Source: three-view drawing plus pictorial views. Frame: mm from the lowest corner of the part. A direction names the side the tool comes from. Round coordinates to 2 decimals unless told otherwise and drop trailing zeros. Order: outer loops, then holes, each group sorted by start corner. A loop starts at its lowest first (then second) coordinate and runs counter-clockwise, first axis right, second up. Notation, with made-up numbers: (-18.5, 49.25) -> (28.5, 49.25) arc R21 cw to (28.5, 70.25) -> close; hole circle Ø5 at (6, 29.5). An arc over 180 degrees is marked (long way). Answer as CSV lines item,"result". Start each with the question number.
1) Section query A-A, the plane y = 78.5. Output: boundary loops of the cut face in (x, z).
2) Section query D-D, the plane z = 10. State how many separate pieces and enclosed holes the cut face has, and give its area (3 significant figures).
3) Section query C-C, the plane y = 61. Output: boundary loops of the cut face in (x, z), and give its area (3 significant figures).
4) Line query: L1, parallel to Z at x = 33.5, y = 3; L2, parallel to Z at x = 113.7, y = 78.5; L3, parallel to X at y = 45.5, z = 13.25. Output: solid intervals per line, ascending.
5) Access query for the marked faces 1, 2, 3 and 4. Directions: +Z, -Z, +X, -X, +Y, -Y. A direction counts if a zero-diameter tool reaches every point of the face in a straight line with its end or side. Return the directions, or none.
6) First-contact query: P1, Ø6, axis at x = 9.5, z = 10, coming from the -Y side; P2, Ø3.5, axis at y = 12.5, z = 10.5, coming from the +X side; P3, Ø3.5, axis at x = 83.5, z = 15, coming from the +Y side. Flat tips, straight axial feed; report the tip coordinate or a pass-through.
7) Section query B-B, the plane x = 33.5. Output: boundary loops of the cut face in (y, z).
8) Mould query, pull axis X, two halves, no side actions, for the marked faces 5, 6, 7 and 8. Classes: +X half, -X half, draft (parallel to the pull), parting line (faces both ways), or undercut.
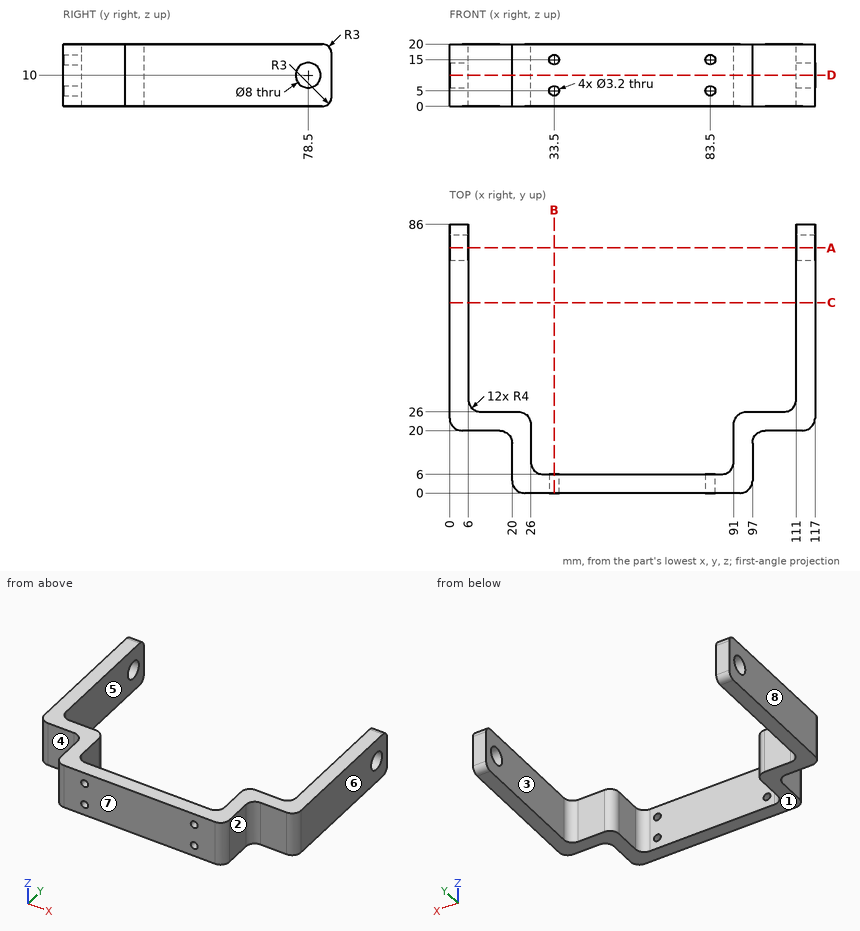
Findings:
1,outline,"(0, 0) -> (6, 0) -> (6, 6) -> (0, 6) -> close; (0, 14) -> (6, 14) -> (6, 20) -> (0, 20) -> close; (111, 0) -> (117, 0) -> (117, 6) -> (111, 6) -> close; (111, 14) -> (117, 14) -> (117, 20) -> (111, 20) -> close"
2,separate pieces,"3"
2,enclosed holes,"0"
2,area,"1,570 mm^2"
3,outline,"(0, 0) -> (6, 0) -> (6, 20) -> (0, 20) -> close; (111, 0) -> (117, 0) -> (117, 20) -> (111, 20) -> close"
3,area,"240 mm^2"
4,L1,"z = 0 to 3.4, 6.6 to 13.4, 16.6 to 20"
4,L2,"z = 0 to 6, 14 to 20"
4,L3,"x = 0 to 6, 111 to 117"
5,face 1,"-Z, +X, -X, +Y, -Y"
5,face 2,"+Z, -Z, +X, -Y"
5,face 3,"+Z, -Z, +Y"
5,face 4,"+Z, -Z, -X, -Y"
6,P1,"stops at y = 20"
6,P2,"stops at x = 97"
6,P3,"stops at y = 6"
7,outline,"(0, 0) -> (6, 0) -> (6, 3.4) -> (0, 3.4) -> close; (0, 6.6) -> (6, 6.6) -> (6, 13.4) -> (0, 13.4) -> close; (0, 16.6) -> (6, 16.6) -> (6, 20) -> (0, 20) -> close"
8,face 5,"undercut"
8,face 6,"+X half"
8,face 7,"draft"
8,face 8,"-X half"
